Autodesk Inventor part; units mm, degrees
ref_plane "YZ Plane" through (0, 0, 0) normal (1, 0, 0) x (0, 1, 0)
ref_plane "XZ Plane" through (0, 0, 0) normal (0, 1, 0) x (-1, 0, 0)
ref_plane "XY Plane" through (0, 0, 0) normal (0, 0, 1) x (1, 0, 0)
sketch "Szkic1" plane through (0, 0, 0) normal (0, 1, 0) x (-1, 0, 0)
  circle A0 centre (0, 0) radius 12.5
  dimension "d0" = 25
extrude "Wyciągnięcie proste1" add sketch "Szkic1" along normal blind 56
sketch "Szkic2" plane through (0, 56, 0) normal (0, 1, 0) x (1, 0, 0)
  circle A0 centre (0, 0) radius 2
  dimension "d3" = 4
extrude "Wyciągnięcie proste2" add sketch "Szkic2" along normal blind 12
sketch "Szkic3" plane through (0, 56, 0) normal (0, 1, 0) x (1, 0, 0)
  circle A0 centre (0, 0) radius 3.5
  dimension "d6" = 7
extrude "Wyciągnięcie proste3" add sketch "Szkic3" along normal blind 2
sketch "Szkic4" plane through (0, 0, 0) normal (0, -1, 0) x (1, 0, 0)
  circle A0 centre (0, 0) radius 2
  circle A1 centre (0, 0) radius 4
  circle A2 centre (0, 0) radius 12.5
  dimension "d9" = 8
extrude "Wyciągnięcie proste4" cut sketch "Szkic4" against normal blind 2 contours A2
sketch "Szkic5" plane through (0, 2, 0) normal (0, -1, 0) x (1, 0, 0)
  line L0 (-9, -4) -> (9, -4)
  line L1 (9, -4) -> (9, 4)
  line L2 (9, 4) -> (-9, 4)
  line L3 (-9, 4) -> (-9, -4)
  circle A0 centre (0, 0) radius 4
  circle A1 centre (0, 0) radius 12.5
  dimension "d12" = 9
  dimension "d13" = 18
extrude "Wyciągnięcie proste5" cut sketch "Szkic5" against normal blind 5
fillet "Zaokrąglenie1" radius 2 4 edges at (-9, 4.5, 4) (-9, 4.5, -4) (9, 4.5, 4) (9, 4.5, -4)
properties part number "Silnik_SKUA"
Can you work these out from the model? Positions are in its coordinate system, mm. A direction names the side the tool comes from. Round coordinates to 2 decimals unless told otherwise and drop trailing zeros. Write each loop counter-clockwise with the first axis right and the second up, starting at its lowest first coordinate (ties: lowest second). Pieces come first, ordered by that corner, then holes. Notation, with made-up numbers: (-17.5, 58.25) -> (11.5, 58.25) arc R23 cw to (11.5, 87.25) -> close; hole circle Ø4 at (-26, 20.25). An arc over 180 degrees is marked (long way). Use one line per item in the form item = value. Start each with the question number.
Q1. I'm going to push flat-ended pins straight in: P1, Ø1.2, axis at y = 4, z = 0, coming from the +X side; P2, Ø10, axis at x = 7, z = -7.5, coming from the +Y side; P3, Ø3, axis at x = -6.5, y = 25.5, coming from the +Z side. Where does each tip first touch, or does it pass through?
Q2. Imagine slicing it at C-C (y = 61). Please give me the cut outline in (x, z).
Q3. Imagine slicing it at D-D (x = -5.5). Please give me the cut outline in (y, z), then the cut area to 3 significant figures.
Q4. Imagine slicing it at B-B (x = -1). Please give me the cut outline in (y, z).
Q5. Which directions (+Z, -Z, +X, -X, +Y, -Y) give clear straight access to the entire face, cutting with the end or side of a thin tool? Please do faces 1 (the face through (-8.4, 4.54, -3.43)), 2 (the face through (0, 63, -2)), 3 (the face through (-0.867, 0.986, -3.905)), 4 (the face through (9, 4, 0)), 5 (the face through (8.4, 4.54, 3.43)).
Q6. Imagine slicing it at A-A (z = 0). Please give me the cut outline in (x, y), then the cut area to 4 significant figures.
Q7. If I drill on probe 1 along Y at (x, z) = (-11.25, 0.5); probe 2 along Y at (x, z) = (-2, -3.5); probe 3 along X at (y, z) = (37, 6.5), over which ranges is the centre line in solid material (lowest first)? Write a range as [from, to].
Worked out:
q1.P1 = 9
q1.P2 = 56
q1.P3 = 11.46
q2.outline = circle Ø4 at (0, 0)
q3.outline = (2, -4) -> (7, -4) -> (7, -11.22) -> (56, -11.22) -> (56, 11.22) -> (7, 11.22) -> (7, 4) -> (2, 4) -> close
q3.area = 1,140 mm^2
q4.outline = (0, -3.87) -> (2, -3.87) -> (2, -4) -> (7, -4) -> (7, -12.46) -> (56, -12.46) -> (56, -3.35) -> (58, -3.35) -> (58, -1.73) -> (68, -1.73) -> (68, 1.73) -> (58, 1.73) -> (58, 3.35) -> (56, 3.35) -> (56, 12.46) -> (7, 12.46) -> (7, 4) -> (2, 4) -> (2, 3.87) -> (0, 3.87) -> close
q5.face_1 = -Z, -X, -Y
q5.face_2 = +Y
q5.face_3 = -Y
q5.face_4 = +Z, -Z, +X, -Y
q5.face_5 = +Z, +X, -Y
q6.outline = (-12.5, 7) -> (-9, 7) -> (-9, 2) -> (-4, 2) -> (-4, 0) -> (4, 0) -> (4, 2) -> (9, 2) -> (9, 7) -> (12.5, 7) -> (12.5, 56) -> (3.5, 56) -> (3.5, 58) -> (2, 58) -> (2, 68) -> (-2, 68) -> (-2, 58) -> (-3.5, 58) -> (-3.5, 56) -> (-12.5, 56) -> close
q6.area = 1,385 mm^2
q7.probe_1 = [7, 56]
q7.probe_2 = [2, 56]
q7.probe_3 = [-10.68, 10.68]
